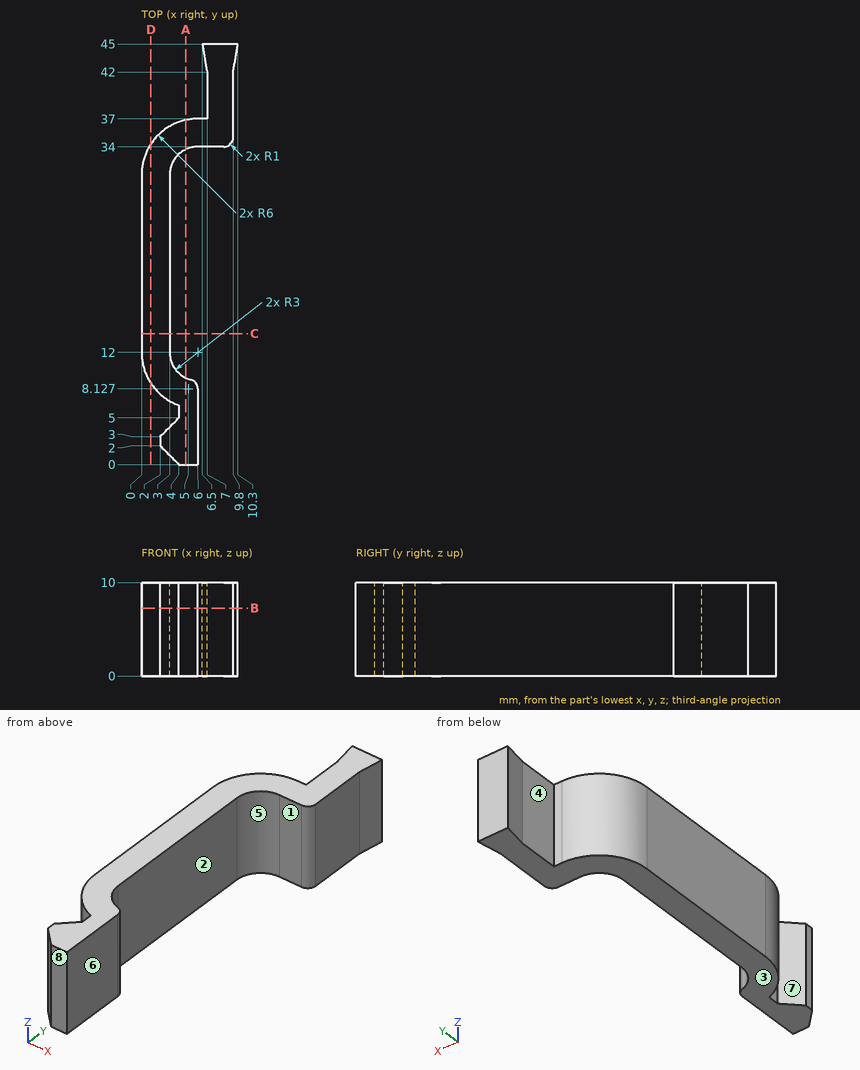
Can you work these out from the drawing? Everything is in mm from the part's minimum corner. A direction names the side the tool comes from. Give positions to 0.01 mm unless a question says otherwise; leave off trailing zeros. Loops run counter-clockwise (first coordinate to the right, second up) from the corner with the lowest first, then second, coordinate; pieces in that order, holes last. Notation, with made-up numbers: (20, 70.5) -> (32, 70.5) arc R27 cw to (32, 91.5) -> close; hole circle Ø2 at (-24, 87.25). An arc over 180 degrees is marked (long way). Return JSON: item names as keys, results as strings.
Q1. I need wall thicknesses on probe 1 along X at (y, z) = (14, 6.5); probe 2 along X at (y, z) = (42, 8.5); probe 3 along Y at (x, z) = (7.5, 6.5). Which ranges of each line are inside material? Lowest first, please.
Checks:
{"probe 1": "x = 0 to 3", "probe 2": "x = 7 to 9.8", "probe 3": "y = 34 to 45"}
Q2. I want a section at C-C, the plane y = 14. List the corners of the cut face in (x, z) for me.
Checks:
{"outline": "(0, 0) -> (3, 0) -> (3, 10) -> (0, 10) -> close"}
Q3. For pin 1 Ø6 at (y, z) = (19.5, 2) entering from +X; pin 2 Ø1.4 at (x, z) = (7.5, 7) entering from -Y; pin 3 Ø3.5 at (y, z) = (38, 7.5) entering from +X, each with a flat end and sliding along its axis, tell me the tip position at first contact or that it passes through.
Checks:
{"pin 1": "stops at x = 3", "pin 2": "stops at y = 34", "pin 3": "stops at x = 9.8"}
Q4. I want a section at B-B, the plane z = 7.25. List the corners of the cut face in (x, y) for me, then the cut area to 3 significant figures.
Checks:
{"outline": "(0, 12) arc R6 ccw to (4, 6.34) -> (4, 5) -> (2, 3) -> (2, 2) -> (4, 0) -> (6, 0) -> (6, 8.13) arc R1 ccw to (5.25, 9.1) arc R3 cw to (3, 12) -> (3, 31) arc R3 cw to (6, 34) -> (8.8, 34) arc R1 ccw to (9.8, 35) -> (9.8, 42) -> (10.3, 45) -> (6.5, 45) -> (7, 42) -> (7, 37) -> (6, 37) arc R6 ccw to (0, 31) -> close", "area": "153 mm2"}
Q5. On a 3-axis mill with a long thin cutter (end or side, diameter ignored), from which of +Z, -Z, +X, -X, +Y, -Y can I reach the whole of each face in a straight line? I mean the marked faces 1, 2, 3 and 4. Say none if no direction works.
Checks:
{"face 1": "+Z, -Z, +X, -Y", "face 2": "+Z, -Z, +X", "face 3": "-Z, +X, -X, +Y, -Y", "face 4": "+Z, -Z, -X"}
Q6. I want a section at D-D, the plane x = 1. List the corners of the cut face in (y, z) for me, then the cut area to 3 significant figures.
Checks:
{"outline": "(8.68, 0) -> (34.32, 0) -> (34.32, 10) -> (8.68, 10) -> close", "area": "256 mm2"}
Q7. We'd pull the mould along Y, two halves only. Please class the marked faces 5, 6, 7 and 8: released by +Y, released by -Y, zero draft, split by the parting line, or undercut.
Checks:
{"face 5": "undercut", "face 6": "zero draft", "face 7": "undercut", "face 8": "released by -Y"}
Q8. I want a section at A-A, the plane x = 4.75. List the corners of the cut face in (y, z) for me, then the cut area to 3 significant figures.
Checks:
{"outline": "(0, 0) -> (9.27, 0) -> (9.27, 10) -> (0, 10) -> close; (33.73, 0) -> (36.87, 0) -> (36.87, 10) -> (33.73, 10) -> close", "area": "124 mm2"}
